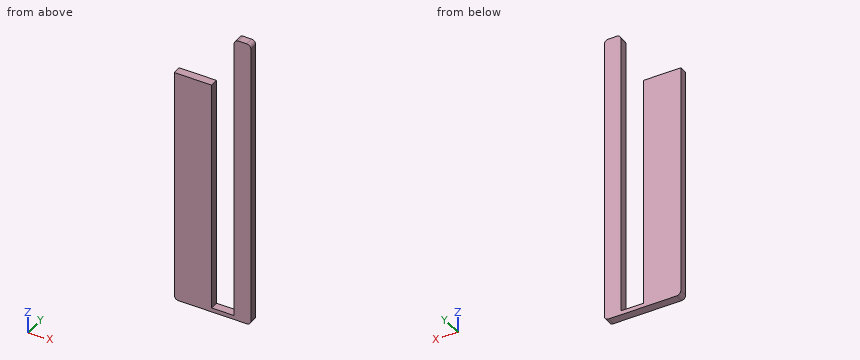
```python
from build123d import *

# Parameters (mm, degrees)
EXTRUDE_1_DEPTH = 2


with BuildPart() as part:
    # ｽｹｯﾁ2 → ﾎﾞｽ - 押し出し1 (new body)
    with BuildSketch(Plane(origin=(0, 0, 0), x_dir=(1, 0, 0), z_dir=(0, 1, 0))):
        with BuildLine():
            Line((0, 0), (9, 0))
            Line((9, 0), (9, 56.55))
            Line((9, 56.55), (14.45, 56.55))
            Line((14.45, 56.55), (14.45, -12.5))
            ThreePointArc((14.45, -12.5), (14.742893219, -13.207106781), (15.45, -13.5))
            Line((15.45, -13.5), (17.45, -13.5))
            ThreePointArc((17.45, -13.5), (18.157106781, -13.207106781), (18.45, -12.5))
            Line((18.45, -12.5), (18.45, 56.55))
            ThreePointArc((18.45, 56.55), (18.157106781, 57.257106781), (17.45, 57.55))
            Line((17.45, 57.55), (1, 57.55))
            ThreePointArc((1, 57.55), (0.292893219, 57.257106781), (0, 56.55))
            Line((0, 56.55), (0, 0))
        make_face()
    extrude(amount=EXTRUDE_1_DEPTH)


solid = part.part
```
For this review, take the finished solid that the model builds, in its own axes (mm). Round coordinates to 2 decimals unless told otherwise and drop trailing zeros. Order: outer loops, then holes, each group sorted by start corner. A loop starts at its lowest first (then second) coordinate and runs counter-clockwise, first axis right, second up. Notation, with made-up numbers: (61.25, 18) -> (104.25, 18) arc R23 ccw to (104.25, 27) -> close; hole circle Ø3 at (66, -13.75). An arc over 180 degrees is marked (long way). Use a Markdown table: item, result.
Item 1: Take a section at A-A (z = -5.5). State the section outline as (x, y) points, plus the area to 3 significant figures.
Resolved:
| item | result |
|---|---|
| outline | (0, 0) -> (9, 0) -> (9, 2) -> (0, 2) -> close; (14.45, 0) -> (18.45, 0) -> (18.45, 2) -> (14.45, 2) -> close |
| area | 26.0 mm² |
Item 2: For line 1 along X through (y, z) = (0.65, -21.5); line 2 along Z through (x, y) = (6, 1.6), list the stretches that pass through material, from the lowest coordinate up. Write a range as [from, to].
Resolved:
| item | result |
|---|---|
| line 1 | x = [0, 9], [14.45, 18.45] |
| line 2 | z = [-57.55, 0] |
Item 3: For pin 1 (0.6 mm diameter, centred on x = 11, y = 1, fed in from +Z), flat-tipped, find the tip position at first contact; note if it passes through.
Resolved:
| item | result |
|---|---|
| pin 1 | stops at z = -56.55 |
Item 4: Take a section at C-C (x = 11.5). State the section outline as (y, z) points, plus the area to 3 significant figures.
Resolved:
| item | result |
|---|---|
| outline | (0, -57.55) -> (2, -57.55) -> (2, -56.55) -> (0, -56.55) -> close |
| area | 2.00 mm² |
Item 5: Take a section at B-B (y = 1.7). State the section outline as (x, z) points, plus the area to 3 significant figures.
Resolved:
| item | result |
|---|---|
| outline | (0, -56.55) arc R1 ccw to (1, -57.55) -> (17.45, -57.55) arc R1 ccw to (18.45, -56.55) -> (18.45, 12.5) arc R1 ccw to (17.45, 13.5) -> (15.45, 13.5) arc R1 ccw to (14.45, 12.5) -> (14.45, -56.55) -> (9, -56.55) -> (9, 0) -> (0, 0) -> close |
| area | 807 mm² |
